Geometry: see drawing. Coordinates: mm, zero at the bounding-box minimum. Round coordinates to 2 decimals unless told otherwise and drop trailing zeros. Loops run counter-clockwise (first coordinate to the right, second up) from the corner with the lowest first, then second, coordinate; pieces in that order, holes last. Notation, with made-up numbers: (-11, 55.25) - (40, 55.25) arc R12 ccw to (40, 66.25) - close; hole circle Ø5 at (-23, -25.75). An arc over 180 degrees is marked (long way). Return JSON: item names as keys, results as strings. Group by question number.
1. Section B-B on y = 4.75. Count the separate pieces of the cut face and the enclosed holes in it, and give its area (3 significant figures).
2. Section C-C on x = 73.5. Return loops of the section in (y, z).
3. First-contact query: pin 1 Ø1.9 at (x, z) = (190, 220) entering from -Y. Flat tip, straight axial feed; report the tip coordinate or a pass-through.
4. Material intervals for probe 1 along Z at (x, y) = (10, 4.75); probe 2 along Z at (x, y) = (100, 7); probe 3 along X at (y, z) = (6.5, 300), sorted ascending.
5. Section A-A on z = 235. Return loops of the section in (x, y), and give its area (3 significant figures).
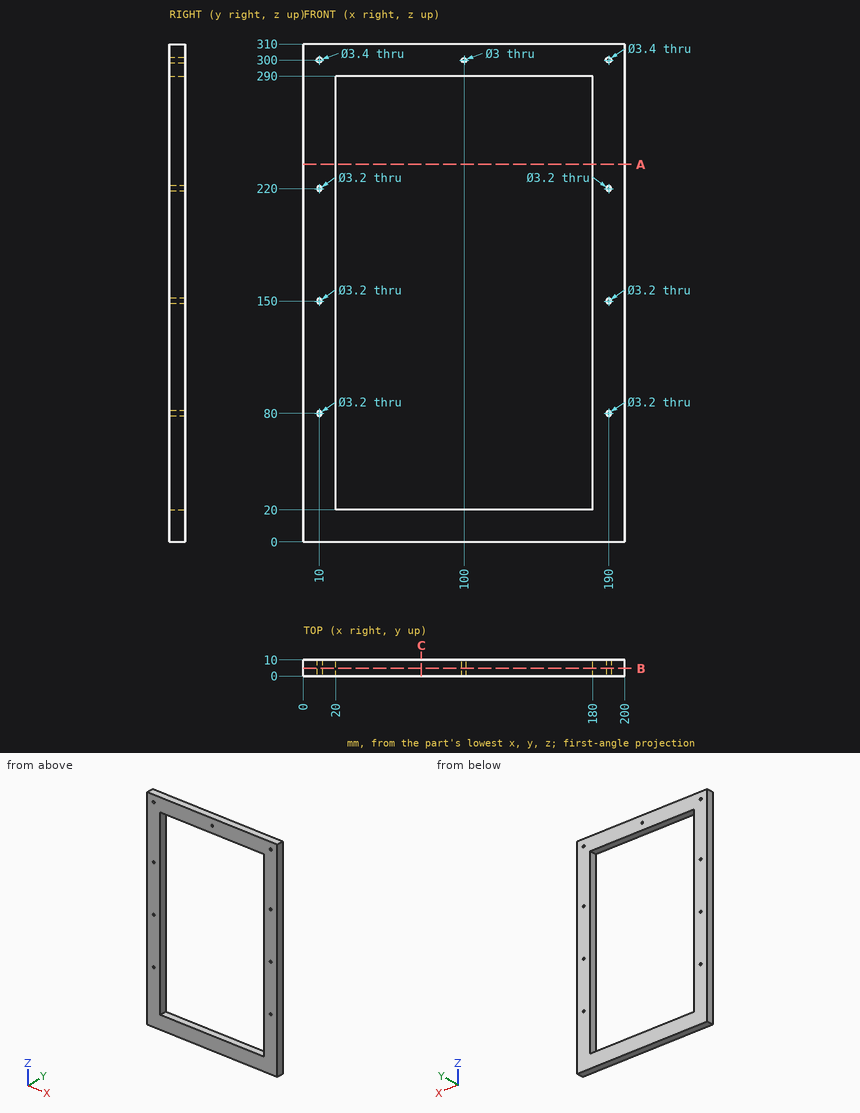
Taken from the geometry:
{
 "1": {"separate pieces": "1", "enclosed holes": "10", "area": "18,700 mm2"},
 "2": {"outline": "(0, 0) - (10, 0) - (10, 20) - (0, 20) - close; (0, 290) - (10, 290) - (10, 310) - (0, 310) - close"},
 "3": {"pin 1": "through"},
 "4": {"probe 1": "0 to 78.4, 81.6 to 148.4, 151.6 to 218.4, 221.6 to 298.3, 301.7 to 310", "probe 2": "0 to 20, 290 to 298.5, 301.5 to 310", "probe 3": "0 to 8.3, 11.7 to 98.5, 101.5 to 188.3, 191.7 to 200"},
 "5": {"outline": "(0, 0) - (20, 0) - (20, 10) - (0, 10) - close; (180, 0) - (200, 0) - (200, 10) - (180, 10) - close", "area": "400 mm2"}
}
